Verification items for the finished model (mm, model axes). Round coordinates to 2 decimals unless told otherwise and drop trailing zeros. Write each loop counter-clockwise with the first axis right and the second up, starting at its lowest first coordinate (ties: lowest second). Pieces come first, ordered by that corner, then holes. Notation, with made-up numbers: (68, 40) -> (94, 40) arc R21 ccw to (94, 72) -> close; hole circle Ø11 at (0.25, 19.25). An arc over 180 degrees is marked (long way). Use CSV: the item, a comma, the result in double quotes.
```python
from build123d import *

# Parameters (mm, degrees)
F0_W     = 71
F0_H     = 57
F0_R     = 8.464637
F1_DEPTH = 2
F2_R     = 2
F4_D     = 2


with BuildPart() as f1:
    # F0 (on Top) → F1 (new body)
    with BuildSketch(Plane.XY):
        Rectangle(F0_W, F0_H)
        with Locations((-12.535542, 0.055034)):
            Circle(F0_R, mode=Mode.SUBTRACT)
        with Locations((12.535542, 0.055034)):
            Circle(F0_R, mode=Mode.SUBTRACT)
    extrude(amount=F1_DEPTH)

    # F2
    f2_edges = [f1.edges().sort_by_distance(p)[0] for p in [
        (-35.5, 28.5, 1),
        (35.5, 28.5, 1),
        (35.5, -28.5, 1),
        (-35.5, -28.5, 1),
    ]]
    fillet(f2_edges, radius=F2_R)

    # F4 (through all)
    with Locations(Plane.XY.offset(2)):
        with Locations((-29.260905, 22.518175), (29.260905, 22.518175), (-29.260905, -22.518175), (29.260905, -22.518175)):
            Hole(F4_D / 2)


solid = f1.part
```
Q1. Go/stop test with a flat-tipped pin: P1, Ø1.8, axis at x = 29.26, y = -22.52, coming from the +Z side. Record where the tip stops, or that it passes through.
Filled in:
P1,"through"
Q2. Mould release check, pull along Y, two halves, no side actions. Record for faces 1 (the cylindrical face through (-30.215, 22.819, 0.986)), 2 (the flat face through (0, -28.5, 1)), 3 (the cylindrical face through (-34.93, 27.9, 1.01)): released by +Y, released by -Y, zero draft, split by the parting line, or undercut.
Filled in:
face 1,"undercut"
face 2,"released by -Y"
face 3,"released by +Y"
Q3. Material ranges on L1, parallel to Y at x = 13, z = 1.5; L2, parallel to X at y = 2, z = 0.3; L3, parallel to X at y = -2.5, z = 1.6, recorded low to high.
Filled in:
L1,"-28.5 to -8.4, 8.51 to 28.5"
L2,"-35.5 to -20.77, -4.3 to 4.3, 20.77 to 35.5"
L3,"-35.5 to -20.61, -4.47 to 4.47, 20.61 to 35.5"
Q4. Section check A-A (x = -5). Record the cut outline in (y, z), plus the area to 3 significant figures.
Filled in:
outline,"(-28.5, 0) -> (-3.8, 0) -> (-3.8, 2) -> (-28.5, 2) -> close; (3.91, 0) -> (28.5, 0) -> (28.5, 2) -> (3.91, 2) -> close"
area,"98.6 mm²"
Q5. Section check C-C (z = 1.15). Record the cut outline in (x, y).
Filled in:
outline,"(-35.5, -26.5) arc R2 ccw to (-33.5, -28.5) -> (33.5, -28.5) arc R2 ccw to (35.5, -26.5) -> (35.5, 26.5) arc R2 ccw to (33.5, 28.5) -> (-33.5, 28.5) arc R2 ccw to (-35.5, 26.5) -> close; hole circle Ø2 at (-29.26, -22.52); hole circle Ø2 at (-29.26, 22.52); hole circle Ø16.93 at (-12.54, 0.06); hole circle Ø16.93 at (12.54, 0.06); hole circle Ø2 at (29.26, -22.52); hole circle Ø2 at (29.26, 22.52)"
Q6. Section check D-D (x = 5.5). Record the cut outline in (y, z).
Filled in:
outline,"(-28.5, 0) -> (-4.65, 0) -> (-4.65, 2) -> (-28.5, 2) -> close; (4.76, 0) -> (28.5, 0) -> (28.5, 2) -> (4.76, 2) -> close"
Q7. Section check B-B (x = -29). Record the cut outline in (y, z).
Filled in:
outline,"(-28.5, 0) -> (-23.48, 0) -> (-23.48, 2) -> (-28.5, 2) -> close; (-21.55, 0) -> (21.55, 0) -> (21.55, 2) -> (-21.55, 2) -> close; (23.48, 0) -> (28.5, 0) -> (28.5, 2) -> (23.48, 2) -> close"
